Source: CAD feature listing. Evaluate the final solid. Frame: model axes, mm. A direction names the side the tool comes from. Round coordinates to 2 decimals unless told otherwise and drop trailing zeros. Order: outer loops, then holes, each group sorted by start corner. A loop starts at its lowest first (then second) coordinate and runs counter-clockwise, first axis right, second up. Notation, with made-up numbers: M -2,34 L 32,34 A32 cw 32,73 Z; hole C 2,-8 d8. An arc over 180 degrees is marked long. Use one line per item in the form item = value. Start each with the question number.
Q1. Section B-B (z = -19). Return the cut outline in (x, y).
Q2. Section C-C (x = 0). Return the cut outline in (y, z), plus the area to 3 significant figures.
Q3. Reachability of faces 4 (the flat face through (35, 7, 0)), 5 (the cylindrical face through (60.01, 9.75, -0.44)), 6 (the flat face through (-52, 10, 0)), 7 (the flat face through (-50, 4, 22)), 8 (the flat face through (52, 10, 0)) from +Z, -Z, +X, -X, +Y, -Y: full face, straight path, thin tool, end or side. Return the list, or none.
Q4. Section A-A (y = 6). Give the number of separate pieces and of enclosed holes in the cut face, plus the area to 3 significant figures.
Q5. Contact query for flat-ended pins moving along their axis: pin 1 (6.5 mm diameter, centred on x = -56.5, y = 5.5, fed in from +Z); pin 2 (18 mm diameter, centred on x = 70, z = 0, fed in from +Y); pin 3 (7 mm diameter, centred on x = -31, z = -7, fed in from -Y). Output: stop coordinate, or through.
Q6. Material intervals for probe 1 along Z at (x, y) = (-70, 2.5); probe 2 along X at (y, z) = (2, 1); probe 3 along X at (y, z) = (21, 22), sorted ascending.
Q7. Pull-direction query (Z, two-part tool) for faces 1 (the flat face through (50, 4, -22)), 2 (the flat face through (-31, 15, 0)), 3 (the flat face through (-61, 4, -15)); classes: pulls with the +Z half, pulls with the -Z half, needs draft (parallel to the pull), parting line crosses it, or undercut.
from build123d import *

# Parameters (mm, degrees)
EXTRUDE_1_DEPTH               = 45
EXTRUDE_2_DEPTH               = 10
SKETCH_3_W                    = 15
SKETCH_3_H                    = 10
CUT_EXTRUDE_1_DEPTH           = 20.000000002
EXTRUDE_3_DEPTH               = 15
CUT_EXTRUDE_2_DEPTH           = 0.8
CUT_EXTRUDE_3_DEPTH           = 0.8
CUT_EXTRUDE_4_DEPTH           = 0.8
CUT_EXTRUDE_5_DEPTH           = 0.8
SKETCH_9_W                    = 70.000000048
SKETCH_9_H                    = 30
CUT_EXTRUDE_6_DEPTH           = 15
HOLE_WIZARD_M52_1_D           = 60
HOLE_WIZARD_M12_1_D           = 13.5
HOLE_WIZARD_M12_1_CBORE_D     = 20
HOLE_WIZARD_M12_1_CBORE_DEPTH = 0.5
FILLET_1_R                    = 2


with BuildPart() as part:
    # 草图1 → 凸台-拉伸1 (new body)
    with BuildSketch(Plane.XY.offset(30)):
        with BuildLine():
            Line((-38.729833462, 10), (38.729833462, 10))
            ThreePointArc((38.729833462, 10), (0, 40), (-38.729833462, 10))
        make_face()
    extrude(amount=-EXTRUDE_1_DEPTH)

    # 草图2 → 凸台-拉伸2 (add)
    with BuildSketch(Plane.XZ.offset(-10)):
        with BuildLine():
            Line((-70, 15), (-50, 15))
            Line((-50, 15), (-50, 30))
            Line((-50, 30), (70, 30))
            Line((70, 30), (70, 15))
            ThreePointArc((70, 15), (85, 0), (70, -15))
            Line((70, -15), (-70, -15))
            ThreePointArc((-70, -15), (-85, 0), (-70, 15))
        make_face()
    extrude(amount=EXTRUDE_2_DEPTH)

    # 草图3 → 切除-拉伸1 (cut)
    with BuildSketch(Plane(origin=(70, 0, 0), x_dir=(0, 0, -1), z_dir=(1, 0, 0))):
        with Locations((-22.5, 5)):
            Rectangle(SKETCH_3_W, SKETCH_3_H)
    extrude(amount=-CUT_EXTRUDE_1_DEPTH, mode=Mode.SUBTRACT)

    # 草图4 → 凸台-拉伸3 (add)
    with BuildSketch(Plane(origin=(0, 0, -15), x_dir=(-1, 0, 0), z_dir=(0, 0, -1))):
        with BuildLine():
            Line((-50, 0), (-50, 10))
            Line((-50, 10), (-38.729833462, 10))
            ThreePointArc((-38.729833462, 10), (0, 40), (38.729833462, 10))
            Line((38.729833462, 10), (50, 10))
            Line((50, 10), (50, 0))
            Line((50, 0), (-50, 0))
        make_face()
    extrude(amount=EXTRUDE_3_DEPTH)

    # 草图5 → 切除-拉伸2 (cut)
    with BuildSketch(Plane.XZ):
        with BuildLine():
            Line((49.999999992, 28), (49.999999992, 29.999999996))
            Line((49.999999992, 29.999999996), (47.999999996, 29.999999996))
            ThreePointArc((47.999999996, 29.999999996), (49.414213556, 29.41421356), (49.999999992, 28))
        make_face()
    extrude(amount=-CUT_EXTRUDE_2_DEPTH, mode=Mode.SUBTRACT)

    # 草图6 → 切除-拉伸3 (cut)
    with BuildSketch(Plane.XZ):
        with BuildLine():
            Line((-48.000000004, 29.999999996), (-50, 29.999999996))
            Line((-50, 29.999999996), (-50, 28))
            ThreePointArc((-50, 28), (-49.414213564, 29.41421356), (-48.000000004, 29.999999996))
        make_face()
    extrude(amount=-CUT_EXTRUDE_3_DEPTH, mode=Mode.SUBTRACT)

    # 草图7 → 切除-拉伸4 (cut)
    with BuildSketch(Plane.XZ):
        with BuildLine():
            Line((48, -30), (49.999999996, -30))
            Line((49.999999996, -30), (49.999999996, -28.000000004))
            ThreePointArc((49.999999996, -28.000000004), (49.41421356, -29.414213564), (48, -30))
        make_face()
    extrude(amount=-CUT_EXTRUDE_4_DEPTH, mode=Mode.SUBTRACT)

    # 草图8 → 切除-拉伸5 (cut)
    with BuildSketch(Plane.XZ):
        with BuildLine():
            Line((-49.999999996, -28.000000004), (-49.999999996, -30))
            Line((-49.999999996, -30), (-48, -30))
            ThreePointArc((-48, -30), (-49.41421356, -29.414213564), (-49.999999996, -28.000000004))
        make_face()
    extrude(amount=-CUT_EXTRUDE_5_DEPTH, mode=Mode.SUBTRACT)

    # 草图9 → 切除-拉伸6 (cut)
    with BuildSketch(Plane.XZ):
        Rectangle(SKETCH_9_W, SKETCH_9_H)
    extrude(amount=-CUT_EXTRUDE_6_DEPTH, mode=Mode.SUBTRACT)

    # M52 间隙孔1 (through all)
    with Locations(Plane(origin=(0, 0, -30), x_dir=(-1, 0, 0), z_dir=(0, 0, -1))):
        with Locations((0, 0)):
            Hole(HOLE_WIZARD_M52_1_D / 2)

    # M12 六角头螺栓的柱形沉头孔1 (through all)
    with Locations(Plane(origin=(0, 10, 0), x_dir=(1, 0, 0), z_dir=(0, 1, 0))):
        with Locations((-70, 0), (70, 0)):
            CounterBoreHole(HOLE_WIZARD_M12_1_D / 2, HOLE_WIZARD_M12_1_CBORE_D / 2, HOLE_WIZARD_M12_1_CBORE_DEPTH)

    # 圆角1
    fillet_1_edges = [part.edges().sort_by_distance(p)[0] for p in [
        (-50, 5.4, 30),
        (-50, 10, 22.5),
        (-60, 10, 15),
        (-85, 10, 0),
        (-60, 10, -15),
        (-50, 10, -22.5),
        (-50, 5.4, -30),
        (-44.364916731, 10, 30),
        (38.729833462, 10, 0),
        (-38.729833462, 10, 0),
        (0, 40, 30),
        (44.36491673, 10, 30),
        (-44.364916731, 10, -30),
        (0, 40, -30),
        (44.364916731, 10, -30),
        (49.999999998, 5.4, 30),
        (50, 5.4, -30),
        (49.999999998, 10, 22.5),
        (59.999999999, 10, 15),
        (85, 10, 0),
        (50, 10, -22.5),
        (60, 10, -15),
        (50, 5, -15),
        (-50, 5, -15),
        (-50, 5, 15),
        (49.999999998, 5, 15),
    ]]
    fillet(fillet_1_edges, radius=FILLET_1_R - 0.0001)  # a hair under: the kernel refuses the full size


solid = part.part
Results list:
q1.outline = M -50,0 L -30,0 A30 cw 30,0 L 50,0 L 50,8 A2 ccw 48,10 L 40.25,10 A2 cw 38.33,11.43 A40 ccw -38.33,11.43 A2 cw -40.25,10 L -48,10 A2 ccw -50,8 Z
q2.outline = M 30,-30 L 38,-30 A2 ccw 40,-28 L 40,28 A2 ccw 38,30 L 30,30 Z
q2.area = 598 mm2
q3.face_4 = -Y
q3.face_5 = +Y
q3.face_6 = +Z, -Z, -X, +Y
q3.face_7 = +Z, -X, +Y, -Y
q3.face_8 = +Z, -Z, +X, +Y
q4.separate_pieces = 2
q4.enclosed_holes = 2
q4.area = 3,760 mm2
q5.pin_1 = 15
q5.pin_2 = 9.5
q5.pin_3 = 15
q6.probe_1 = -15 to -6.75, 6.75 to 15
q6.probe_2 = -84.97 to -76.68, -63.32 to -35, 35 to 63.32, 76.68 to 84.97
q6.probe_3 = -34.04 to -21.42, 21.42 to 34.04
q7.face_1 = needs draft
q7.face_2 = undercut
q7.face_3 = pulls with the -Z half
